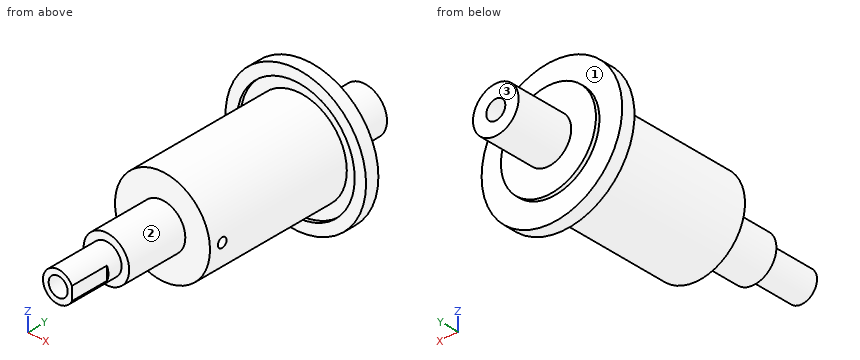
Autodesk Inventor part; units mm, degrees
ref_plane "Work Plane1" through (12.5, 0, 0) normal (1, 0, 0) x (0, 1, 0)
ref_plane "XZ Plane" through (0, 0, 0) normal (0, 1, 0) x (-1, 0, 0)
ref_plane "XY Plane" through (0, 0, 0) normal (0, 0, 1) x (1, 0, 0)
sketch "Sketch1" plane through (0, 0, 0) normal (0, 0, 1) x (1, 0, 0)
  line L0 (0, -17.5) -> (8.5, -17.5)
  line L1 (8.5, -17.5) -> (8.5, 17.5)
  line L2 (8.5, 17.5) -> (0, 17.5)
  line L3 (0, 17.5) -> (0, -17.5)
  line L4 (8.5, 11.5) -> (18.5, 11.5)
  line L5 (18.5, 11.5) -> (18.5, 9)
  line L6 (18.5, 9) -> (8.5, 9)
  line L7 (8.5, 9) -> (8.5, 11.5)
  line L8 (18.5, 9) -> (15.5, 9)
  line L9 (15.5, 9) -> (15.5, 8)
  line L10 (15.5, 8) -> (18.5, 8)
  line L11 (18.5, 8) -> (18.5, 9)
  line L12 (0, -24.5) -> (0, 24.5) construction
  line L13 (8.5, -17.5) -> (12.5, -17.5)
  line L14 (12.5, -17.5) -> (12.5, 9)
  line L15 (12.5, 9) -> (8.5, 9)
  line L16 (8.5, 9) -> (8.5, -17.5)
  line L17 (8.5, 11.5) -> (6, 11.5)
  line L18 (6, 11.5) -> (6, 17.5)
  point P0 (0, 0)
  point P1 (0, 0)
  point P2 (8.5, 9)
  dimension "d0" = 35
  dimension "d1" = 8.5
  dimension "d2" = 10
  dimension "d3" = 2.5
  dimension "d4" = 6
  dimension "d5" = 3
  dimension "d6" = 1
  dimension "d32" = 4
  dimension "d69" = 6
revolve "Revolution1" add sketch "Sketch1" angle 360 about axis through (0, -10, 0) along (0, 1, 0) contours L3 L2 L18 L17 L1 L0 | L1 L6 L14 L13 | L1 L4 L5 L6 | L6 L11 L10 L9
sketch "Sketch3" plane through (0, -17.5, 0) normal (0, -1, 0) x (1, 0, 0)
  circle A0 centre (0, 0) radius 12.5
extrude "Extrusion1" add sketch "Sketch3" along normal blind 12.5
sketch "Sketch4" plane through (0, -30, 0) normal (0, -1, 0) x (1, 0, 0)
  circle A0 centre (0, 0) radius 4
  circle A1 centre (0, 0) radius 12.5
  dimension "d24" = 8
extrude "Extrusion2" add sketch "Sketch4" along normal blind 29.75 contours A0
sketch "Sketch5" plane through (0, 17.5, 0) normal (0, 1, 0) x (1, 0, 0)
  circle A0 centre (0, 0) radius 6
extrude "Extrusion3" add sketch "Sketch5" along normal blind 10
sketch "Sketch6" plane through (0, 11.5, 0) normal (0, 1, 0) x (1, 0, 0)
  circle A0 centre (0, 0) radius 2.621
  circle A1 centre (0, 0) radius 12.5
  circle A2 centre (0, 0) radius 6
  dimension "d29" = 25
extrude "Extrusion4" add sketch "Sketch6" along normal blind 1 contours A0 | A1 | A2
sketch "Sketch7" plane through (0, 27.5, 0) normal (0, 1, 0) x (1, 0, 0)
  point P0 (0, 0)
  point P1 (0, 0)
hole "Hole2" at (0, 27.5, 0) direction (0, -1, 0) diameter 3.242 end through all
sketch "Sketch8" plane through (0, 27.5, 0) normal (0, 1, 0) x (1, 0, 0)
  circle A0 centre (0, 0) radius 2.5
  dimension "d41" = 5
extrude "Extrusion5" cut sketch "Sketch8" against normal blind 10
sketch "Sketch9" plane through (0, -59.75, 0) normal (0, -1, 0) x (1, 0, 0)
  circle A0 centre (0, 0) radius 2.5
  dimension "d44" = 5
extrude "Extrusion6" cut sketch "Sketch9" against normal blind 50
chamfer "Chamfer3" distance 0.5 angle 30 1 edges at (0, -9.75, -1.621) measured on face at (2.1788, -9.75, -0.2646)
chamfer "Chamfer4" distance 0.5 angle 30 1 edges at (0, 17.5, -1.621) measured on face at (2.1788, 17.5, 0.2646)
ref_plane "Work Plane1" through (12.5, 0, 0) normal (1, 0, 0) x (0, 1, 0)
sketch "Sketch10" plane through (12.5, 0, 0) normal (1, 0, 0) x (0, 1, 0)
  line L0 (27.5, -8.5) -> (27.5, 8.5)
  line L1 (-37.3, 0) -> (38.3, 0)
  point P0 (0, 0)
  point P1 (-26.5, 0)
  dimension "d54" = 54
hole "Hole3" at (12.5, -26.5, 0) direction (-1, 0, 0) diameter 2.459 depth 8.8 tip angle 118
sketch "Sketch11" plane through (0, -59.75, 0) normal (0, -1, 0) x (1, 0, 0)
  circle A0 centre (0, 0) radius 2.5
  circle A1 centre (0, 0) radius 4
  line L0 (3.6, -1.7436) -> (3.6, 1.7436)
  point P0 (3.6, 0)
  dimension "d65" = 3.6
extrude "Extrusion7" cut sketch "Sketch11" against normal blind 10 contours A0 | A1 L0 picked at (3.6735, -0.3949)
sketch "Sketch12" plane through (0, -30, 0) normal (0, -1, 0) x (1, 0, 0)
  circle A0 centre (0, 0) radius 6
  circle A1 centre (0, 0) radius 2.5
  dimension "d66" = 12
extrude "Extrusion8" add sketch "Sketch12" along normal blind 16
properties part number "shaft"
Geometry check sheet. Reference: the model listing, model coordinates, mm. Face numbers are marked on the shaded views. A direction names the side the tool comes from. Give positions to 0.01 mm unless a question says otherwise; leave off trailing zeros. Write each loop counter-clockwise with the first axis right and the second up, starting at its lowest first coordinate (ties: lowest second). Pieces come first, ordered by that corner, then holes. Notation, with made-up numbers: M 16.5,7 L 69.5,7 A23 ccw 69.5,17 Z; hole C 16.25,57.5 d10. An arc over 180 degrees is marked long. Answer as CSV lines item,"result". Start each with the question number.
Q1. Section check B-B, the plane z = -14.5. Record the cut outline in (x, y).
Q2. Tool access check on the marked faces 1, 2 and 3. Record the directions out of +Z, -Z, +X, -X, +Y, -Y that give a thin tool (end or side, any length) a straight path to the whole face; none if there is none.
Q3. Section check A-A, the plane y = -11.5. Record the cut outline in (x, z), then the cut area to 3 significant figures.
Q4. Go/stop test with flat-tipped pins: pin 1 (2 mm diameter, centred on x = -4.5, z = 8, fed in from -Y); pin 2 (6 mm diameter, centred on x = 12, z = 0, fed in from +Y); pin 3 (8 mm diameter, centred on y = -44, z = -4.5, fed in from +X). Record where each tip stops, or that it passes through.
Q5. Section check C-C, the plane z = -9.5. Record the cut outline in (x, y), then the cut area to 3 significant figures.
Q6. Material ranges on L1, parallel to Z at x = 0, y = 8.6; L2, parallel to Y at x = 10, z = 0, recorded low to high.
Q7. Section check D-D, the plane z = 8. Record the cut outline in (x, y).
Geometry says:
1,outline,"M -11.49,8 L -5.48,8 L -5.48,9 L 5.48,9 L 5.48,8 L 11.49,8 L 11.49,11.5 L -11.49,11.5 Z"
2,face 1,"+Y"
2,face 2,"-Y"
2,face 3,"+Z, -Z, +X, -X, +Y"
3,outline,"C 0,0 d25; hole C 0,0 d5"
3,area,"471 mm^2"
4,pin 1,"y = -30"
4,pin 2,"y = 12.5"
4,pin 3,"x = 5.98"
5,outline,"M -15.87,8 L -12.25,8 L -12.25,9 L -8.12,9 L -8.12,-30 L 8.12,-30 L 8.12,9 L 12.25,9 L 12.25,8 L 15.87,8 L 15.87,11.5 L 8.12,11.5 L 8.12,12.5 L -8.12,12.5 L -8.12,11.5 L -15.87,11.5 Z"
5,area,"737 mm^2"
6,L1,"-18.5 to -15.5, -12.5 to -1.62, 1.62 to 12.5, 15.5 to 18.5"
6,L2,"-30 to -27.73, -25.27 to 12.5"
7,outline,"M -16.68,8 L -13.28,8 L -13.28,9 L -9.6,9 L -9.6,-30 L 9.6,-30 L 9.6,9 L 13.28,9 L 13.28,8 L 16.68,8 L 16.68,11.5 L 9.6,11.5 L 9.6,12.5 L -9.6,12.5 L -9.6,11.5 L -16.68,11.5 Z"
